```python
from build123d import *

# Parameters (mm, degrees)
F2_DEPTH = 4
F1_R     = 2.6
F3_DEPTH = 5
F4_R     = 1
F6_DEPTH = 4


with BuildPart() as f2:
    # F0 (on Top) → F2 (new body)
    with BuildSketch(Plane.XY):
        with BuildLine():
            Line((39.760675, -6.1935), (1.883808, 5.90006))
            ThreePointArc((1.883808, 5.90006), (-5.905721, 1.865987), (-1.848149, -5.911327))
            Line((-1.848149, -5.911327), (-1.848149, -13.865659))
            Line((-1.848149, -13.865659), (3.065253, -13.865659))
            Line((3.065253, -13.865659), (3.065253, -6.1935))
            Line((3.065253, -6.1935), (39.760675, -6.1935))
        make_face()
    extrude(amount=-F2_DEPTH)

    # F1 (on Top) → F3 (cut)
    with BuildSketch(Plane.XY):
        Circle(F1_R)
    extrude(amount=-F3_DEPTH, mode=Mode.SUBTRACT)

    # F4
    f4_edges = [f2.edges().sort_by_distance(p)[0] for p in [
        (-2.6, 0, 0),
        (-2.6, 0, -4),
    ]]
    fillet(f4_edges, radius=F4_R)

    # F5 (on Top) → F6 (join)
    with BuildSketch(Plane.XY):
        Polygon((-4.70453, 3.279649), (-3.058211, 5.351829), (-7.161808, 10.117297), (-9.131761, 8.420949), (-8.328387, 8.181407), (-8.481963, 7.666345), align=None)
    extrude(amount=-F6_DEPTH)


solid = f2.part
```
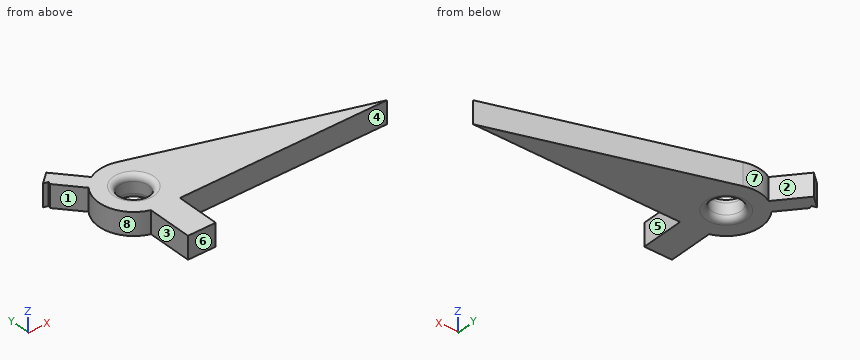
Design review of the part built by this model. Coordinates are the model's own, in mm. Face numbers are marked on the shaded views. A direction names the side the tool comes from. Coordinates: 2 decimals unless noted, no trailing zeros. Write each loop counter-clockwise with the first axis right and the second up, starting at its lowest first coordinate (ties: lowest second). Pieces come first, ordered by that corner, then holes.
1) Mouldability with a two-part tool opening along X and no side actions: class the marked faces 5, 6, 7 and 8 as +X half, -X half, draft (parallel to the pull), parting line (faces both ways), or undercut.
2) Add section B-B (z = -2.35). Write out the cut boundary in (x, y), plus the area to 3 significant figures.
3) Add section D-D (y = -10). Write out the cut boundary in (x, z).
4) Add section C-C (y = 0). Write out the cut boundary in (x, z).
5) To check wall thickness, follow L1, parallel to Y at x = 0, z = -2.55; L2, parallel to X at y = -6.25, z = -0.95; L3, parallel to Y at x = 2, z = -1.3. State the ranges of each line that lie inside material, in increasing order.
6) Machinability: for the marked faces 1, 2, 3 and 4, which of the approach directions +Z, -Z, +X, -X, +Y, -Y give a long, thin tool a straight path to every point of the face, cutting with its end or side? Answer none if there is none.
7) Add section A-A (x = 0). Write out the cut boundary in (y, z).
8) Insertion check: pin 1 (1.2 mm diameter, centred on y = -11, z = -2, fed in from -X); pin 2 (6 mm diameter, centred on x = 8.5, y = -0.5, fed in from +Z); pin 3 (2 mm diameter, centred on y = 5, z = -2.5, fed in from -X). Each pin has a flat end and moves straight along its axis. Give the tip position at first contact, or say it passes through.
Check result:
1. face 5: +X half
1. face 6: draft
1. face 7: undercut
1. face 8: -X half
2. outline: (-9.13, 8.42) - (-8.33, 8.18) - (-8.48, 7.67) - (-5.01, 3.64) arc R6.19 ccw to (-1.85, -5.91) - (-1.85, -13.87) - (3.07, -13.87) - (3.07, -6.19) - (39.76, -6.19) - (1.88, 5.9) arc R6.19 ccw to (-3.08, 5.37) - (-7.16, 10.12) - close; hole circle Ø5.2 at (0, 0)
2. area: 345 mm2
3. outline: (-1.85, -4) - (3.07, -4) - (3.07, 0) - (-1.85, 0) - close
4. outline: (-6.19, -4) - (-3.6, -4) arc R1 ccw to (-2.6, -3) - (-2.6, -1) arc R1 ccw to (-3.6, 0) - (-6.19, 0) - close; (2.6, -3) arc R1 ccw to (3.6, -4) - (20.36, -4) - (20.36, 0) - (3.6, 0) arc R1 ccw to (2.6, -1) - close
5. L1: y = -13.87 to -2.6, 2.6 to 6.19
5. L2: x = -1.85 to 3.07
5. L3: y = -13.87 to -1.66, 1.66 to 5.86
6. face 1: +Z, -Z, -X
6. face 2: +Z, -Z, +Y
6. face 3: +Z, -Z, -X, -Y
6. face 4: +Z, -Z, +X, -Y
7. outline: (-13.87, -4) - (-3.6, -4) arc R1 ccw to (-2.6, -3) - (-2.6, -1) arc R1 ccw to (-3.6, 0) - (-13.87, 0) - close; (2.6, -3) arc R1 ccw to (3.6, -4) - (6.19, -4) - (6.19, 0) - (3.6, 0) arc R1 ccw to (2.6, -1) - close
8. pin 1: stops at x = -1.85
8. pin 2: stops at z = 0
8. pin 3: stops at x = -7.05
